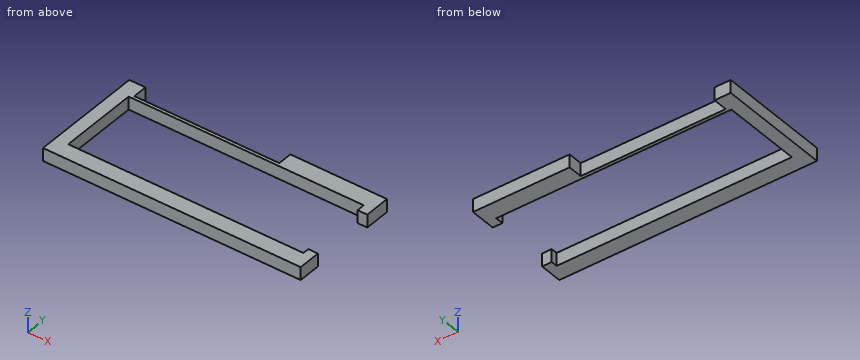
Autodesk Fusion 360 part; units mm, degrees
sketch "Sketch1" plane through (0, 0, 0) normal (0, 0, 1) x (1, 0, 0)
  line L0 (0, 0) -> (0, 35)
  line L1 (0, 35) -> (80, 35)
  line L2 (80, 35) -> (80, 27)
  line L3 (80, 27) -> (77, 27)
  line L4 (77, 27) -> (77, 29.5)
  line L5 (77, 29.5) -> (4, 29.5)
  line L6 (4, 29.5) -> (4, 5)
  line L7 (4, 5) -> (77, 5)
  line L8 (77, 5) -> (77, 7)
  line L9 (77, 7) -> (80, 7)
  line L10 (80, 7) -> (80, 0)
  line L11 (80, 0) -> (0, 0)
  line L12 (4.2162, 35) -> (5, 35)
  line L13 (4, 32) -> (4.2162, 32)
  line L14 (5, 35) -> (50, 35)
  line L15 (50, 35) -> (50, 30.5)
  line L16 (50, 30.5) -> (5, 30.5)
  line L17 (5, 30.5) -> (5, 35)
  dimension "d3" = 35
  dimension "d4" = 5
  dimension "d5" = 5.5
  dimension "d6" = 3
  dimension "d7" = 3
  dimension "d8" = 8
  dimension "d9" = 7
  dimension "d10" = 4
  dimension "d11" = 80
  dimension "d12" = 80
  dimension "d13" = 45
  dimension "d14" = 5
  dimension "d15" = 4.5
extrude "Extrude1" add sketch "Sketch1" along normal blind 4 contours L0 L1 L2 L3 L4 L5 L6 L7 L8 L9 L10 L11 L12 L15 L16 L17
The model under review builds one solid part; all positions refer to its coordinate system, in mm. Give positions to 0.01 mm unless a question says otherwise; leave off trailing zeros. Loops run counter-clockwise (first coordinate to the right, second up) from the corner with the lowest first, then second, coordinate; pieces in that order, holes last. Notation, with made-up numbers: (35.25, 30.5) -> (64.25, 30.5) arc R10 ccw to (64.25, 42.5) -> close; hole circle Ø10 at (-28, 61). An arc over 180 degrees is marked (long way). Use CSV: the item, a comma, the result in double quotes.
1. For P1, Ø8, axis at x = 44.5, y = 12.5, coming from the -Z side; P2, Ø1.2, axis at y = 22.5, z = 2, coming from the +X side; P3, Ø1.2, axis at x = 38, z = 1, coming from the +Y side, all flat-tipped, find the tip position at first contact; note any pin that passes through.
Result:
P1,"passes through"
P2,"stops at x = 4"
P3,"stops at y = 30.5"
2. Consider section C-C, the plane y = 26. Write out the cut boundary in (x, z).
Result:
outline,"(0, 0) -> (4, 0) -> (4, 4) -> (0, 4) -> close"
3. Consider section A-A, the plane x = 63. Write out the cut boundary in (y, z).
Result:
outline,"(0, 0) -> (5, 0) -> (5, 4) -> (0, 4) -> close; (29.5, 0) -> (35, 0) -> (35, 4) -> (29.5, 4) -> close"
4. To check wall thickness, follow probe 1 along Y at (x, z) = (30.5, 3.1); probe 2 along Y at (x, z) = (58.5, 3.4); probe 3 along X at (y, z) = (33, 1.1). State the ranges of each line that lie inside material, in increasing order. Write a range as from..to.
Result:
probe 1,"y = 0..5, 29.5..30.5"
probe 2,"y = 0..5, 29.5..35"
probe 3,"x = 0..5, 50..80"
5. Consider section D-D, the plane x = 22. Write out the cut boundary in (y, z).
Result:
outline,"(0, 0) -> (5, 0) -> (5, 4) -> (0, 4) -> close; (29.5, 0) -> (30.5, 0) -> (30.5, 4) -> (29.5, 4) -> close"
6. Consider section B-B, the plane z = 2.85. Write out the cut boundary in (x, y).
Result:
outline,"(0, 0) -> (80, 0) -> (80, 7) -> (77, 7) -> (77, 5) -> (4, 5) -> (4, 29.5) -> (77, 29.5) -> (77, 27) -> (80, 27) -> (80, 35) -> (50, 35) -> (50, 30.5) -> (5, 30.5) -> (5, 35) -> (0, 35) -> close"
